Input: part model. Units: mm. Frame: model coordinates. Give positions to 0.01 mm unless a question says otherwise; leave off trailing zeros. Write each loop counter-clockwise with the first axis right and the second up, starting at its lowest first coordinate (ties: lowest second). Pieces come first, ordered by that corner, then holes. Notation, with made-up numbers: (49, -36.75) - (98, -36.75) arc R11 cw to (98, -29.75) - close; hole circle Ø7 at (-33, -10). An arc over 180 degrees is marked (long way). Use a Markdown table: item, result. Add a question column.
1. Mould query, pull axis Z, two halves, no side actions, for faces 1 (the cylindrical face through (3.616, 1.862, 3.921)), 2 (the flat face through (3.859, 2, 0)), 3 (the cylindrical face through (-1.71, 1.82, -0.38)), 4 (the cylindrical face through (-5.498, 1.838, 0.164)). Classes: released by +Z, released by -Z, zero draft, split by the parting line, or undercut.
2. Section query B-B, the plane y = 1.85. Return loops of the section in (x, z).
3. Pin query (flat end, axial travel): pin 1 (2 mm diameter, centred on x = 1.5, y = 2, fed in from -Z); pin 2 (1 mm diameter, centred on x = -2.5, z = 3, fed in from -Y). Return the tip coordinate at first contact, or that it passes through.
4. Material intervals for probe 1 along X at (y, z) = (2.5, 0); probe 2 along Z at (x, y) = (-4.5, 2.35); probe 3 along X at (y, z) = (0.75, -2), sorted ascending.
5. Section query A-A, the plane z = 0. Return loops of the section in (x, y).
```python
from build123d import *

# Parameters (mm, degrees)
CROQUIS1_R              = 1.75
SALIENTE_EXTRUIR1_DEPTH = 3.7
REDONDEO1_R             = 2
REDONDEO2_R             = 1


with BuildPart() as part:
    # Croquis1 → Saliente-Extruir1 (new body)
    with BuildSketch(Plane(origin=(0, 0, 0), x_dir=(1, 0, 0), z_dir=(0, 1, 0))):
        with BuildLine():
            Line((3.858987824, 3.918955597), (3.858987824, -3.918955597))
            ThreePointArc((3.858987824, -3.918955597), (-5.5, 0), (3.858987824, 3.918955597))
        make_face()
        with Locations(Location((0, 0, 0), (0, 0, 270))):
            Circle(CROQUIS1_R, mode=Mode.SUBTRACT)
    extrude(amount=SALIENTE_EXTRUIR1_DEPTH)

    # Redondeo1
    redondeo1_edges = [part.edges().sort_by_distance(p)[0] for p in [
        (3.858987824, 1.85, -3.918955597),
        (3.858987824, 1.85, 3.918955597),
    ]]
    fillet(redondeo1_edges, radius=REDONDEO1_R)

    # Redondeo2
    redondeo2_edges = [part.edges().sort_by_distance(p)[0] for p in [
        (3.858987824, 0, 0),
        (3.858987824, 3.7, 0),
        (-5.5, 0, 0),
        (3.60892461, 0, -3.933855699),
        (3.60892461, 0, 3.933855699),
        (-5.5, 3.7, 0),
        (3.60892461, 3.7, -3.933855699),
        (3.60892461, 3.7, 3.933855699),
    ]]
    fillet(redondeo2_edges, radius=REDONDEO2_R)


solid = part.part
```
Result sheet:
| question | item | result |
|---|---|---|
| 1 | face 1 | released by +Z |
| 1 | face 2 | zero draft |
| 1 | face 3 | undercut |
| 1 | face 4 | split by the parting line |
| 2 | outline | (2.92, -4.66) arc R2 ccw to (3.86, -2.97) - (3.86, 2.97) arc R2 ccw to (2.92, 4.66) arc R5.5 ccw (long way) to start; hole circle Ø3.5 at (0, 0) |
| 3 | pin 1 | stops at z = -5.48 |
| 3 | pin 2 | stops at y = 0 |
| 4 | probe 1 | x = -5.5 to -1.75, 1.75 to 3.86 |
| 4 | probe 2 | z = -3.16 to 3.16 |
| 4 | probe 3 | x = -5.09 to 3.83 |
| 5 | outline | (-5.5, 1) arc R1 ccw to (-4.5, 0) - (-1.75, 0) - (-1.75, 3.7) - (-4.5, 3.7) arc R1 ccw to (-5.5, 2.7) - close; (1.75, 0) - (2.86, 0) arc R1 ccw to (3.86, 1) - (3.86, 2.7) arc R1 ccw to (2.86, 3.7) - (1.75, 3.7) - close |
